Design review of the part built by this model. Coordinates are the model's own, in mm. A direction names the side the tool comes from. Give positions to 0.01 mm unless a question says otherwise; leave off trailing zeros. Write each loop counter-clockwise with the first axis right and the second up, starting at its lowest first coordinate (ties: lowest second). Pieces come first, ordered by that corner, then holes. Notation, with made-up numbers: (44.25, -32) -> (86.25, -32) arc R18 ccw to (86.25, -17) -> close; hole circle Ø11 at (57.5, 34.25). An arc over 180 degrees is marked (long way). Return JSON: item names as keys, results as strings. Group by question number.
from build123d import *

# Parameters (mm, degrees)
F0_R     = 2.032
F0_R_2   = 2.0955
F0_R_3   = 1.905
F1_DEPTH = 5.715
F3_DEPTH = 1.524
F5_DEPTH = 1.524
F7_DEPTH = 40.64


with BuildPart() as f1:
    # F0 (on Top) → F1 (new body)
    with BuildSketch(Plane.XY):
        with BuildLine():
            Line((42.979039, -11.196153), (35.252589, 23.228599))
            ThreePointArc((35.252589, 23.228599), (22.99115, 39.586517), (2.617796, 41.274961))
            Line((2.617796, 41.274961), (-35.34082, 27.858045))
            Line((-35.34082, 27.858045), (-35.34082, 22.778045))
            Line((-35.34082, 22.778045), (-43.27832, 22.778045))
            Line((-43.27832, 22.778045), (-43.27832, -23.576955))
            Line((-43.27832, -23.576955), (-35.34082, -23.576955))
            Line((-35.34082, -23.576955), (-35.34082, -28.192097))
            Line((-35.34082, -28.192097), (-23.079528, -42.787694))
            Line((-23.079528, -42.787694), (-2.65018, -42.787694))
            Line((-2.65018, -42.787694), (37.631817, -22.502827))
            ThreePointArc((37.631817, -22.502827), (42.249864, -17.769064), (42.979039, -11.196153))
        make_face()
        with Locations((-18.264627, -37.707694)):
            Circle(F0_R, mode=Mode.SUBTRACT)
        with Locations((-8.739627, -37.707694)):
            Circle(F0_R, mode=Mode.SUBTRACT)
        with Locations((-39.30957, -17.861955)):
            Circle(F0_R_2, mode=Mode.SUBTRACT)
        with Locations((-3.20238, -11.133077)):
            Circle(F0_R_3, mode=Mode.SUBTRACT)
        with Locations((-11.414669, -5.413778)):
            Circle(F0_R_3, mode=Mode.SUBTRACT)
        with Locations((36.516652, -14.728804)):
            Circle(F0_R, mode=Mode.SUBTRACT)
        with Locations((-39.30957, 17.063045)):
            Circle(F0_R_2, mode=Mode.SUBTRACT)
        with Locations((-15.07797, 20.994581)):
            Circle(F0_R_2, mode=Mode.SUBTRACT)
        Polygon((26.502235, 22.29995), (3.192089, -10.990389), (-3.830092, -6.073405), (-7.836523, -11.795182), (-10.437331, -9.974077), (-6.4309, -4.2523), (-13.453081, 0.664684), (9.857066, 33.955024), (16.879247, 29.03804), (20.885678, 34.759817), (23.486486, 32.938711), (19.480055, 27.216934), align=None, mode=Mode.SUBTRACT)
        with Locations((16.266104, 34.118518)):
            Circle(F0_R, mode=Mode.SUBTRACT)
        with Locations((24.46385, 28.378394)):
            Circle(F0_R, mode=Mode.SUBTRACT)
    extrude(amount=-F1_DEPTH)

    # F2 (on face) → F3 (join)
    with BuildSketch(Plane.XY):
        with BuildLine():
            Line((-35.34082, 22.778045), (-35.34082, -23.576955))
            Line((-35.34082, -23.576955), (-35.34082, -28.192097))
            Line((-35.34082, -28.192097), (-29.210174, -35.489896))
            Line((-29.210174, -35.489896), (-27.265349, -33.85611))
            Line((-27.265349, -33.85611), (-32.80082, -27.266796))
            Line((-32.80082, -27.266796), (-32.80082, -23.576955))
            Line((-32.80082, -23.576955), (-32.80082, 22.778045))
            Line((-32.80082, 22.778045), (-32.80082, 26.061838))
            Line((-32.80082, 26.061838), (3.464267, 38.880157))
            ThreePointArc((3.464267, 38.880157), (21.761995, 37.363731), (32.774246, 22.672349))
            Line((32.774246, 22.672349), (40.500696, -11.752404))
            ThreePointArc((40.500696, -11.752404), (39.953697, -16.683147), (36.489417, -20.234232))
            Line((36.489417, -20.234232), (0.186785, -38.515204))
            Line((0.186785, -38.515204), (0.186785, -41.359079))
            Line((0.186785, -41.359079), (37.631817, -22.502827))
            ThreePointArc((37.631817, -22.502827), (42.249864, -17.769064), (42.979039, -11.196153))
            Line((42.979039, -11.196153), (35.252589, 23.228599))
            ThreePointArc((35.252589, 23.228599), (22.99115, 39.586517), (2.617796, 41.274961))
            Line((2.617796, 41.274961), (-35.34082, 27.858045))
            Line((-35.34082, 27.858045), (-35.34082, 22.778045))
        make_face()
    extrude(amount=F3_DEPTH)

    # F4 (on face) → F5 (join)
    with BuildSketch(Plane.XY):
        Polygon((-28.899134, -31.911285), (-27.265349, -33.85611), (0.186785, -33.85611), (0.186785, -38.515204), (2.726785, -37.236132), (2.726785, -31.31611), (-28.19065, -31.31611), align=None)
    extrude(amount=F5_DEPTH)

    # F6 (on face) → F7 (join)
    with BuildSketch(Plane(origin=(19.196518, 27.415469, 0), x_dir=(0.819152, -0.573576, 0), z_dir=(-0.573576, -0.819152, 0))):
        Polygon((-19.021366, 0), (-11.401366, 0), (-11.401366, 7.62), align=None)
        Polygon((8.918634, 7.62), (8.918634, 0), (16.538634, 0), align=None)
    extrude(amount=F7_DEPTH)


solid = f1.part
Q1. Take a section at A-A, the plane z = 3.5. Give the boundary of the cut face in (x, y), plus the area to 3 significant figures.
Q2. Mouldability with a two-part tool opening along Y and no side actions: class faces 1 (the face through (-13, -42.788, -3)), 2 (the face through (21.5, 30.1, -2.8)), 3 (the face through (-39, 0, 0)) as +Y half, -Y half, draft (parallel to the pull), parting line (faces both ways), or undercut.
Q3. Tool access review of faces 4 (the face through (15.01, 5.89, -2.82)), 5 (the face through (-39, 22.778, -3)), 6 (the face through (-15, -38, 0)), 7 (the face through (28.19, 21.12, 2.17)): name each direction out of +Z, -Z, +X, -X, +Y, -Y from which nothing blocks a thin tool from reaching the whole face with its end or side.
Q4. Take a section at D-D, the plane z = -4.25. Count the separate pieces of the cut face and the enclosed holes in it, plus the area to 3 significant figures.
Q5. Take a section at C-C, the plane x = 25.5. Give the boundary of the cut face in (y, z) (3 decimals), plus the area to 3 significant figures.
Q6. For L1, parallel to Y at x = -8.5, z = -1; L2, parallel to Z at x = 32, y = 0 (3 decimals); L3, parallel to Y at x = -6.5, z = 0.75, list the stretches that pass through material, from the lowest coordinate up. Write a range as from..to.
Q7. Insertion check: pin 1 (5 mm diameter, centred on x = -11.41, y = -5.41, fed in from -Z) (3 decimals); pin 2 (1.7 mm diameter, centred on y = -36, z = 0.5, fed in from -X); pin 3 (1.7 mm diameter, centred on y = -1, z = 0.5, fed in from +X); pin 4 (3 mm diameter, centred on x = -15, z = -2, fed in from +Y). Each pin has a flat end and moves straight along its axis. Give the tip position at first contact, or say it passes through.
Final values:
{
 "1": {"outline": "(-16.83, 3.03) -> (-13.45, 0.66) -> (9.86, 33.96) -> (6.48, 36.32) -> close; (3.19, -10.99) -> (6.57, -13.35) -> (29.88, 19.94) -> (26.5, 22.3) -> close", "area": "335 mm²"},
 "2": {"face 1": "-Y half", "face 2": "undercut", "face 3": "draft"},
 "3": {"face 4": "+Z, -Z", "face 5": "+Z, -Z, -X, +Y", "face 6": "+Z, -Y", "face 7": "+Z"},
 "4": {"separate pieces": "1", "enclosed holes": "11", "area": "4,730 mm²"},
 "5": {"outline": "(-28.612, -5.715) -> (20.869, -5.715) -> (20.869, 7.62) -> (7.584, 0) -> (-25.768, 0) -> (-25.768, 1.524) -> (-28.612, 1.524) -> close; (23.002, -5.715) -> (26.63, -5.715) -> (26.63, 0) -> (23.002, 0) -> close; (30.126, -5.715) -> (37.997, -5.715) -> (37.997, 1.524) -> (34.768, 1.524) -> (34.768, 0) -> (30.126, 0) -> close", "area": "408 mm²"},
 "6": {"L1": "y = -42.79..-39.73, -35.69..-11.33, -7.21..-2.8, 7.74..37.35", "L2": "z = -5.715..0", "L3": "y = -33.86..-31.32, 10.59..22.57, 35.36..38.05"},
 "7": {"pin 1": "stops at z = -5.715", "pin 2": "stops at x = -29.5", "pin 3": "stops at x = 40.88", "pin 4": "stops at y = 35.58"}
}
